Source: three-view drawing plus pictorial views. Frame: mm from the lowest corner of the part. A direction names the side the tool comes from. Round coordinates to 2 decimals unless told otherwise and drop trailing zeros. Loops run counter-clockwise (first coordinate to the right, second up) from the corner with the lowest first, then second, coordinate; pieces in that order, holes last. Notation, with made-up numbers: (30, 41) -> (78, 41) arc R15 cw to (78, 49) -> close; hole circle Ø11 at (57.25, 33.5). An arc over 180 degrees is marked (long way). Put each result on its own line as item: value. Start each with the question number.
1. Cut plane C-C (z = 6.75). Return the cut outline in (x, y), then the cut area to 3 significant figures.
2. Draft query along X for the marked faces 4, 5, 6 and 7. Return one class per face: pulls with the +X half, pulls with the -X half, needs draft (parallel to the pull), parting line crosses it, or undercut.
3. Contact query for flat-ended pins moving along their axis: pin 1 (1.5 mm diameter, centred on x = 17, z = 5, fed in from -Y); pin 2 (3.5 mm diameter, centred on y = 19, z = 3.5, fed in from -X); pin 3 (6 mm diameter, centred on x = 59, y = 11.5, fed in from +Z); pin 4 (1.8 mm diameter, centred on x = 3.5, z = 7.5, fed in from +Y). Output: stop coordinate, or through.
4. Cut plane D-D (x = 55). Return the cut outline in (y, z).
5. Cut plane A-A (x = 22.5). Return the cut outline in (y, z).
6. Set-up query: the marked faces 1, 2 and 3. Return all of +Z, -Z, +X, -X, +Y, -Y with unobstructed straight access to the full face (end or side cutting, diameter ignored); none if empty.
7. Cut plane B-B (y = 17). Return the cut outline in (x, z), then the cut area to 3 significant figures.
8. Material intervals for L1, parallel to Y at x = 15.5, z = 9.5; L2, parallel to Y at x = 85, z = 2.75; L3, parallel to X at y = 29.5, z = 7.75, sorted ascending.
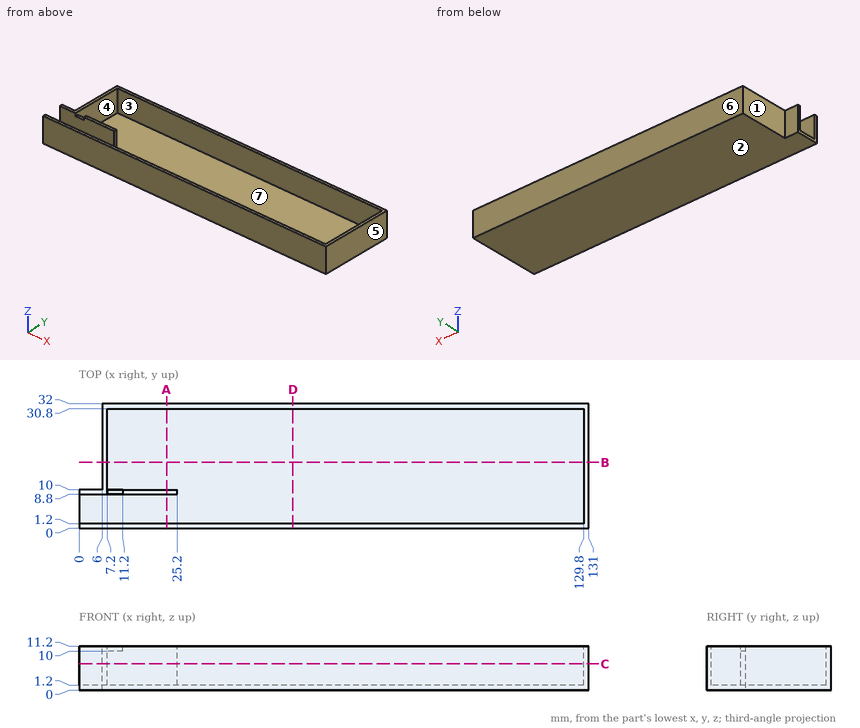
Solution:
1. outline: (0, 0) -> (131, 0) -> (131, 32) -> (6, 32) -> (6, 10) -> (0, 10) -> (0, 8.8) -> (25.2, 8.8) -> (25.2, 10) -> (7.2, 10) -> (7.2, 30.8) -> (129.8, 30.8) -> (129.8, 1.2) -> (0, 1.2) -> close
1. area: 398 mm^2
2. face 4: undercut
2. face 5: pulls with the +X half
2. face 6: needs draft
2. face 7: undercut
3. pin 1: stops at y = 0
3. pin 2: stops at x = 6
3. pin 3: stops at z = 1.2
3. pin 4: stops at y = 10
4. outline: (0, 0) -> (32, 0) -> (32, 11.2) -> (30.8, 11.2) -> (30.8, 1.2) -> (1.2, 1.2) -> (1.2, 11.2) -> (0, 11.2) -> close
5. outline: (0, 0) -> (32, 0) -> (32, 11.2) -> (30.8, 11.2) -> (30.8, 1.2) -> (10, 1.2) -> (10, 11.2) -> (8.8, 11.2) -> (8.8, 1.2) -> (1.2, 1.2) -> (1.2, 11.2) -> (0, 11.2) -> close
6. face 1: +Z, -Z, -X, +Y
6. face 2: -Z, +X, -X, +Y, -Y
6. face 3: +Z
7. outline: (6, 0) -> (131, 0) -> (131, 11.2) -> (129.8, 11.2) -> (129.8, 1.2) -> (7.2, 1.2) -> (7.2, 11.2) -> (6, 11.2) -> close
7. area: 174 mm^2
8. L1: y = 0 to 1.2, 8.8 to 10, 30.8 to 32
8. L2: y = 0 to 1.2, 30.8 to 32
8. L3: x = 6 to 7.2, 129.8 to 131
